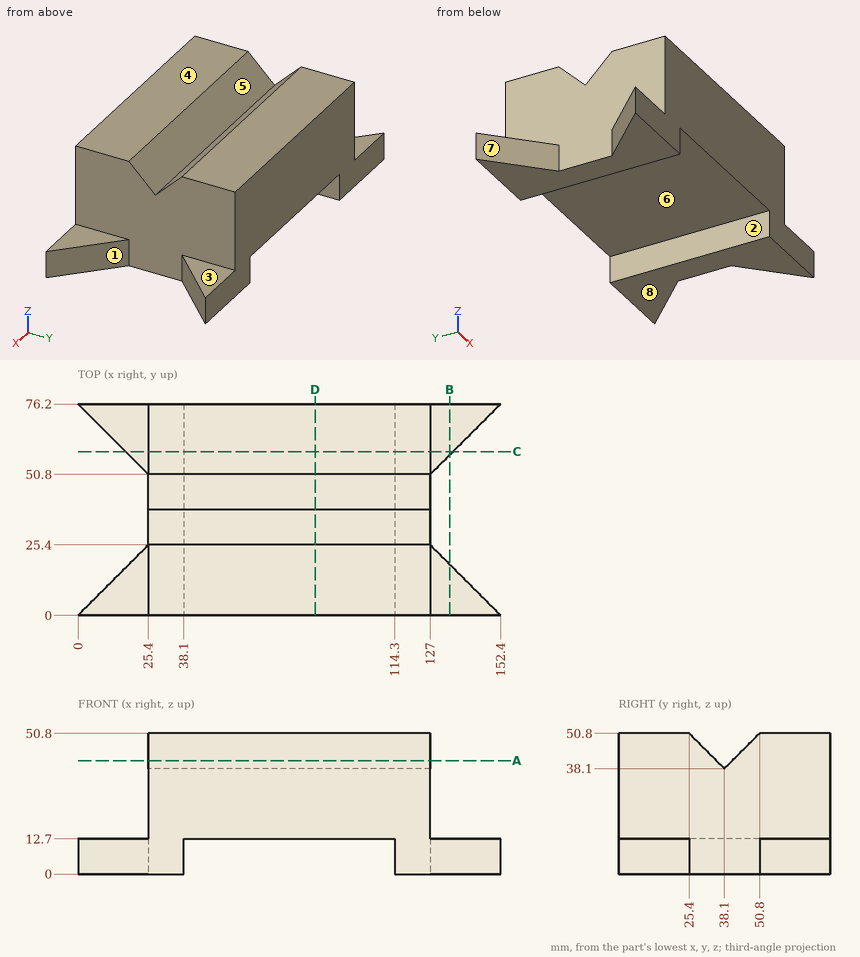
Drawing for the job (mm, zero at the part's lowest x, y, z). A direction names the side the tool comes from. Give positions to 0.01 mm unless a question says otherwise; leave off trailing zeros. Loops run counter-clockwise (first coordinate to the right, second up) from the corner with the lowest first, then second, coordinate; pieces in that order, holes last.
1) 3-axis set-ups, long thin cutter, end or side, ignore diameter. For the marked faces 1, 2, 3, 4 and 5: which of +Z, -Z, +X, -X, +Y, -Y reach the whole face in a straight line?
Values follow:
face 1: +Z, -Z, +X
face 2: -Z, +Y, -Y
face 3: +Z, +X, +Y, -Y
face 4: +Z, +X, -X, +Y, -Y
face 5: +Z, +X, -X
2) Band-saw the part on C-C on y = 59. List the corners of the cut face in (x, z), then the cut area to 3 significant figures.
Values follow:
outline: (17.2, 0) - (38.1, 0) - (38.1, 12.7) - (114.3, 12.7) - (114.3, 0) - (135.2, 0) - (135.2, 12.7) - (127, 12.7) - (127, 50.8) - (25.4, 50.8) - (25.4, 12.7) - (17.2, 12.7) - close
area: 4,400 mm2
3) Probe line 1 along X through (y, z) = (47, 7); line 2 along Z through (x, y) = (102, 62.5); line 3 along X through (y, z) = (65, 34.5). List the from-to ranges inside material, lowest first.
Values follow:
line 1: x = 25.4 to 38.1, 114.3 to 127
line 2: z = 12.7 to 50.8
line 3: x = 25.4 to 127
4) Drop flat-ended pins along their axis: P1, Ø3, axis at x = 106.5, y = 38.5, coming from the -Z side; P2, Ø20.5, axis at x = 11, y = 9, coming from the +Z side; P3, Ø6, axis at y = 57.5, z = 32.5, coming from the -X side. Give the stop position or say it passes through.
Values follow:
P1: stops at z = 12.7
P2: stops at z = 12.7
P3: stops at x = 25.4
5) Band-saw the part on D-D on x = 85.5. List the corners of the cut face in (y, z), then the cut area to 3 significant figures.
Values follow:
outline: (0, 12.7) - (76.2, 12.7) - (76.2, 50.8) - (50.8, 50.8) - (38.1, 38.1) - (25.4, 50.8) - (0, 50.8) - close
area: 2,740 mm2
6) Band-saw the part on B-B on x = 134. List the corners of the cut face in (y, z), then the cut area to 3 significant figures.
Values follow:
outline: (0, 0) - (18.4, 0) - (18.4, 12.7) - (0, 12.7) - close; (57.8, 0) - (76.2, 0) - (76.2, 12.7) - (57.8, 12.7) - close
area: 467 mm2
7) Two-plate mould, pull along X, no slides. Class the marked faces 6, 7 and 8: released by +X, released by -X, zero draft, split by the parting line, or undercut.
Values follow:
face 6: undercut
face 7: released by -X
face 8: zero draft
8) Band-saw the part on A-A on z = 41. List the corners of the cut face in (x, y).
Values follow:
outline: (25.4, 0) - (127, 0) - (127, 35.2) - (25.4, 35.2) - close; (25.4, 41) - (127, 41) - (127, 76.2) - (25.4, 76.2) - close
